For this review, use the dimensioned drawing (mm, ordinates from the lowest corner) and the shaded views. A direction names the side the tool comes from. Coordinates: 2 decimals unless noted, no trailing zeros. Write each loop counter-clockwise with the first axis right and the second up, starting at its lowest first coordinate (ties: lowest second). Pieces come first, ordered by that corner, then holes. Notation, with made-up numbers: M -15,-36.5 L 30,-36.5 A27 ccw 30,-4.5 Z; hole C 69,81 d4. An arc over 180 degrees is marked long. Return JSON: item names as keys, results as strings.
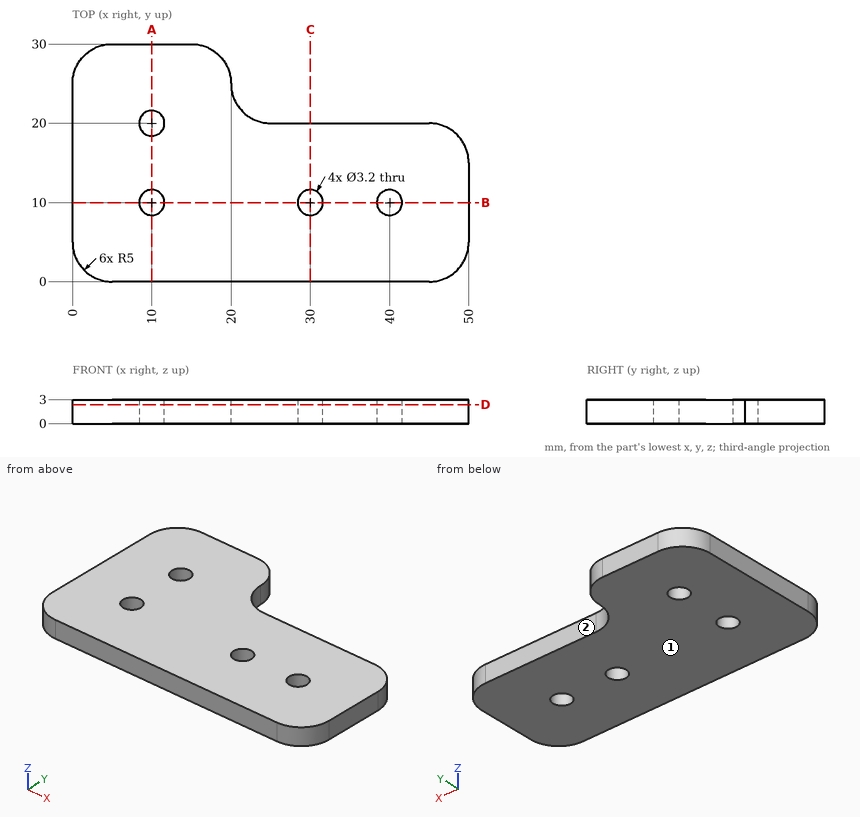
1. We need section C-C (x = 30). State the section outline as (y, z) points.
Checks:
{"outline": "M 0,0 L 8.4,0 L 8.4,3 L 0,3 Z; M 11.6,0 L 20,0 L 20,3 L 11.6,3 Z"}
2. We need section B-B (y = 10). State the section outline as (x, z) points.
Checks:
{"outline": "M 0,0 L 8.4,0 L 8.4,3 L 0,3 Z; M 11.6,0 L 28.4,0 L 28.4,3 L 11.6,3 Z; M 31.6,0 L 38.4,0 L 38.4,3 L 31.6,3 Z; M 41.6,0 L 50,0 L 50,3 L 41.6,3 Z"}
3. Wall thickness on L1, parallel to Y at x = 10, z = 2.3; L2, parallel to Y at x = 40, z = 1.9; L3, parallel to Y at x = 26, z = 2.4: over which ranges is each line inside the solid? List them lowest first. Write a range as from..to.
Checks:
{"L1": "0..8.4, 11.6..18.4, 21.6..30", "L2": "0..8.4, 11.6..20", "L3": "0..20"}
4. For the marked faces 1 and 2, list the 3-axis set-ups (+Z, -Z, +X, -X, +Y, -Y) from which the entire face can be reached by the end or side of a thin tool; tool diameter is ignored.
Checks:
{"face 1": "-Z, +X, -X, +Y, -Y", "face 2": "+Z, -Z, +X, +Y"}
5. We need section A-A (x = 10). State the section outline as (y, z) points, plus the area to 3 significant figures.
Checks:
{"outline": "M 0,0 L 8.4,0 L 8.4,3 L 0,3 Z; M 11.6,0 L 18.4,0 L 18.4,3 L 11.6,3 Z; M 21.6,0 L 30,0 L 30,3 L 21.6,3 Z", "area": "70.8 mm2"}
6. We need section D-D (z = 2.4). Give the number of separate pieces and of enclosed holes in the cut face, plus the area to 3 significant figures.
Checks:
{"separate pieces": "1", "enclosed holes": "4", "area": "1,150 mm2"}
7. Clearance check with flat-ended pins moving along their axes: pin 1 Ø6 at (x, y) = (41, 25.5) entering from -Z; pin 2 Ø1 at (y, z) = (20, 1.5) entering from +X. State where each tip first meets the part, or that it passes through.
Checks:
{"pin 1": "through", "pin 2": "x = 47.18"}
